```python
from build123d import *

# Parameters (mm, degrees)
BASE_FLANGE1_DEPTH            = 1.7366
EDGE_FLANGE1_STRIP_W          = 8.4196
EDGE_FLANGE1_STRIP_H          = 1.7366
EDGE_FLANGE1_STRIP_CUT_DEPTH  = 600.1
EDGE_FLANGE1_RELIEF_W         = 9.2879
EDGE_FLANGE1_RELIEF_H         = 0.8683
EDGE_FLANGE1_RELIEF_CUT_DEPTH = 1.7366
EDGE_FLANGE1_DEPTH            = 600.1
EDGE_FLANGE2_STRIP_W          = 8.4196
EDGE_FLANGE2_STRIP_H          = 1.7366
EDGE_FLANGE2_STRIP_CUT_DEPTH  = 544.6
EDGE_FLANGE2_RELIEF_W         = 9.2879
EDGE_FLANGE2_RELIEF_H         = 0.8683
EDGE_FLANGE2_RELIEF_CUT_DEPTH = 1.7366
EDGE_FLANGE2_DEPTH            = 544.6


# Sheet-metal steps are written as plain solids
with BuildPart() as part:
    # Sketch1 → Base-Flange1 (new body)
    with BuildSketch(Plane(origin=(0, 0, 0), x_dir=(1, 0, 0), z_dir=(0, 1, 0))):
        Polygon((-105.270941838, 479.5), (-105.270941838, 469.5), (-120.270941838, 469.5), (-120.270941838, 139.5), (-135.270941838, 139.5), (-135.270941838, -469.5), (-120.270941838, -469.5), (-105.270941838, -469.5), (-105.270941838, -479.5), (104.429058162, -479.5), (104.429058162, -469.5), (114.429058162, -469.5), (114.429058162, 469.5), (104.429058162, 469.5), (104.429058162, 479.5), align=None)
    extrude(amount=-BASE_FLANGE1_DEPTH)

    # Edge-Flange1 strip (across the edge) → Edge-Flange1 strip cut (cut)
    with BuildSketch(Plane(origin=(-135.270941838, -1.7366, 469.1), x_dir=(1, 0, 0), z_dir=(0, 0, -1))):
        with Locations((-3.4732, -0.8683)):
            Rectangle(EDGE_FLANGE1_STRIP_W, EDGE_FLANGE1_STRIP_H)
    extrude(amount=EDGE_FLANGE1_STRIP_CUT_DEPTH, mode=Mode.SUBTRACT)

    # Edge-Flange1 relief (on the sheet) → Edge-Flange1 relief cut (cut)
    with BuildSketch(Plane(origin=(-134.534341838, -1.7366, 469.1), x_dir=(1, 0, 0), z_dir=(0, -1, 0))):
        with Locations((-3.77565, 0.43415)):
            Rectangle(EDGE_FLANGE1_RELIEF_W, EDGE_FLANGE1_RELIEF_H)
        with Locations((-3.77565, -600.53415)):
            Rectangle(EDGE_FLANGE1_RELIEF_W, EDGE_FLANGE1_RELIEF_H)
    extrude(amount=-EDGE_FLANGE1_RELIEF_CUT_DEPTH, mode=Mode.SUBTRACT)

    # Edge-Flange1 section (across the edge) → Edge-Flange1 (add)
    with BuildSketch(Plane(origin=(-135.270941838, -1.7366, 469.1), x_dir=(1, 0, 0), z_dir=(0, 0, -1))):
        with BuildLine():
            Line((-1.7366, 0.7366), (-1.7366, 42))
            Line((-1.7366, 42), (0, 42))
            Line((0, 42), (0, 0.7366))
            ThreePointArc((0, 0.7366), (0.215745145, 0.215745145), (0.7366, 0))
            Line((0.7366, 0), (0.7366, -1.7366))
            ThreePointArc((0.7366, -1.7366), (-1.012216491, -1.012216491), (-1.7366, 0.7366))
        make_face()
    extrude(amount=EDGE_FLANGE1_DEPTH)

    # Edge-Flange2 strip (across the edge) → Edge-Flange2 strip cut (cut)
    with BuildSketch(Plane(origin=(-137.007541838, -43.7366, -75.5), x_dir=(0, 1, 0), z_dir=(0, 0, 1))):
        with Locations((-3.4732, -0.8683)):
            Rectangle(EDGE_FLANGE2_STRIP_W, EDGE_FLANGE2_STRIP_H)
    extrude(amount=EDGE_FLANGE2_STRIP_CUT_DEPTH, mode=Mode.SUBTRACT)

    # Edge-Flange2 relief (on the sheet) → Edge-Flange2 relief cut (cut)
    with BuildSketch(Plane(origin=(-137.007541838, -43, -75.5), x_dir=(0, 1, 0), z_dir=(-1, 0, 0))):
        with Locations((-3.77565, 0.43415)):
            Rectangle(EDGE_FLANGE2_RELIEF_W, EDGE_FLANGE2_RELIEF_H)
    extrude(amount=-EDGE_FLANGE2_RELIEF_CUT_DEPTH, mode=Mode.SUBTRACT)

    # Edge-Flange2 section (across the edge) → Edge-Flange2 (add)
    with BuildSketch(Plane(origin=(-137.007541838, -43.7366, -75.5), x_dir=(0, 1, 0), z_dir=(0, 0, 1))):
        with BuildLine():
            Line((-1.7366, 0.7366), (-1.7366, 40))
            Line((-1.7366, 40), (0, 40))
            Line((0, 40), (0, 0.7366))
            ThreePointArc((0, 0.7366), (0.215745145, 0.215745145), (0.7366, 0))
            Line((0.7366, 0), (0.7366, -1.7366))
            ThreePointArc((0.7366, -1.7366), (-1.012216491, -1.012216491), (-1.7366, 0.7366))
        make_face()
    extrude(amount=EDGE_FLANGE2_DEPTH)


solid = part.part
```
Verification items for the finished model (mm, model axes). A direction names the side the tool comes from. Round coordinates to 2 decimals unless told otherwise and drop trailing zeros. Order: outer loops, then holes, each group sorted by start corner. A loop starts at its lowest first (then second) coordinate and runs counter-clockwise, first axis right, second up. Notation, with made-up numbers: (78.5, -36.5) - (132.5, -36.5) arc R18 ccw to (132.5, -8.5) - close; hole circle Ø1 at (22, 6.5). An arc over 180 degrees is marked (long way). Use CSV: the item, a comma, the result in double quotes. Start each with the question number.
1) Section check B-B, the plane x = 91. Record the cut outline in (y, z), plus the area to 3 significant figures.
2) Section check C-C, the plane y = -23.5. Record the cut outline in (x, z), plus the area to 3 significant figures.
3) Go/stop test with flat-tipped pins: P1, Ø19.5, axis at x = -150, z = 330, coming from the +Y side; P2, Ø6, axis at x = 4, z = 35.5, coming from the +Y side; P3, Ø0.5, axis at x = 107.5, y = -0.5, coming from the +Z side; P4, Ø1.9, axis at x = -136.5, z = -95.5, coming from the -Y side. Record where each tip stops, or that it passes through.
4) Section check A-A, the plane z = 212. Record the cut outline in (x, y).
5) Access from +Z, -Z, +X, -X, +Y, -Y to the whole of each face (thin tool, end or side, straight path). Record for faces 1 (the flat face through (-12, -1.737, -7)), 2 (the flat face through (-12, 0, -7)), 3 (the flat face through (-158, -43.737, 193)).
6) Thickness scan on L1, parallel to X at y = -42, z = -104.5; L2, parallel to Y at x = -160.5, z = 269.5; L3, parallel to Y at x = 25, z = 53.5. Record the ranges inside material, lowest first.
Answers:
1,outline,"(-1.74, -479.5) - (0, -479.5) - (0, 479.5) - (-1.74, 479.5) - close"
1,area,"1,670 mm²"
2,outline,"(-137.01, -131) - (-135.27, -131) - (-135.27, 469.1) - (-137.01, 469.1) - close"
2,area,"1,040 mm²"
3,P1,"stops at y = -43.74"
3,P2,"stops at y = 0"
3,P3,"stops at z = 469.5"
3,P4,"stops at y = -43.74"
4,outline,"(-177.01, -45.47) - (-137.74, -45.47) arc R2.47 ccw to (-135.27, -43) - (-135.27, -2.47) arc R0.74 cw to (-134.53, -1.74) - (114.43, -1.74) - (114.43, 0) - (-134.53, 0) arc R2.47 ccw to (-137.01, -2.47) - (-137.01, -43) arc R0.74 cw to (-137.74, -43.74) - (-177.01, -43.74) - close"
5,face 1,"+Z, -Z, +X, -Y"
5,face 2,"+Z, -Z, +X, -X, +Y"
5,face 3,"+Z, -Z, -X, +Y"
6,L1,"x = -137.01 to -135.27"
6,L2,"y = -45.47 to -43.74"
6,L3,"y = -1.74 to 0"
